```python
from build123d import *

# Parameters (mm, degrees)
SKETCH_1_W      = 50
SKETCH_1_H      = 20
SKETCH_1_R      = 1.6
EXTRUDE_1_DEPTH = 3


with BuildPart() as part:
    # 草图1 → 凸台-拉伸1 (new body)
    with BuildSketch(Plane.XY):
        with Locations((25, -10)):
            Rectangle(SKETCH_1_W, SKETCH_1_H)
        with Locations((45, -5)):
            Circle(SKETCH_1_R, mode=Mode.SUBTRACT)
        with Locations(Location((45, -15, 0), (0, 0, 180))):
            Circle(SKETCH_1_R, mode=Mode.SUBTRACT)
        with Locations((35, -15)):
            Circle(SKETCH_1_R, mode=Mode.SUBTRACT)
        with Locations(Location((35, -5, 0), (0, 0, 180))):
            Circle(SKETCH_1_R, mode=Mode.SUBTRACT)
        with Locations((5, -6.25)):
            Circle(SKETCH_1_R, mode=Mode.SUBTRACT)
        with Locations(Location((5, -13.75, 0), (0, 0, 180))):
            Circle(SKETCH_1_R, mode=Mode.SUBTRACT)
        with Locations((15, -13.75)):
            Circle(SKETCH_1_R, mode=Mode.SUBTRACT)
        with Locations(Location((15, -6.25, 0), (0, 0, 180))):
            Circle(SKETCH_1_R, mode=Mode.SUBTRACT)
    extrude(amount=EXTRUDE_1_DEPTH)


solid = part.part
```
Model file for the job. Use its own axes, mm. Give positions to 0.01 mm unless a question says otherwise; leave off trailing zeros. Order: outer loops, then holes, each group sorted by start corner. A loop starts at its lowest first (then second) coordinate and runs counter-clockwise, first axis right, second up.
1) Saw through at C-C, the plane x = 5. Write the cut outline in (y, z).
2) Saw through at B-B, the plane y = -4. Write the cut outline in (x, z).
3) Wall check: probe 1 along Y at (x, z) = (5, 1.2); probe 2 along Y at (x, z) = (35, 1.5); probe 3 along X at (y, z) = (-12.5, 2.7). Give the ranges that are in metal, low to high.
4) Saw through at A-A, the plane z = 0.9. Count the separate pieces of the cut face and the enclosed holes in it, then the cut area to 3 significant figures.
5) Mould opens along X. For faces 1 (the flat face through (50, -10, 1)), 2 (the flat face through (0, -10, 1)), 3 (the flat face through (25, -10, 0)), 4 (the cylindrical face through (16.6, -6.3, 1.5)) say: +X half, -X half, draft (parallel to the pull), parting line (faces both ways), or undercut.
Computed:
1. outline: (-20, 0) - (-15.35, 0) - (-15.35, 3) - (-20, 3) - close; (-12.15, 0) - (-7.85, 0) - (-7.85, 3) - (-12.15, 3) - close; (-4.65, 0) - (0, 0) - (0, 3) - (-4.65, 3) - close
2. outline: (0, 0) - (33.75, 0) - (33.75, 3) - (0, 3) - close; (36.25, 0) - (43.75, 0) - (43.75, 3) - (36.25, 3) - close; (46.25, 0) - (50, 0) - (50, 3) - (46.25, 3) - close
3. probe 1: y = -20 to -15.35, -12.15 to -7.85, -4.65 to 0
3. probe 2: y = -20 to -16.6, -13.4 to -6.6, -3.4 to 0
3. probe 3: x = 0 to 4, 6 to 14, 16 to 50
4. separate pieces: 1
4. enclosed holes: 8
4. area: 936 mm2
5. face 1: +X half
5. face 2: -X half
5. face 3: draft
5. face 4: undercut
